from build123d import *

# Parameters (mm, degrees)
F0_R     = 12.5
F2_DEPTH = 236.5
F4_DEPTH = 4


with BuildPart() as f2:
    # F0 (on Right) → F2 (new body, symmetric)
    with BuildSketch(Plane.YZ):
        Circle(F0_R)
    extrude(amount=F2_DEPTH, both=True)

    # F3 (on offset) → F4 (cut)
    with BuildSketch(Plane.XY.offset(12.5)):
        with BuildLine():
            ThreePointArc((-136.5, 4), (-140.5, 0), (-136.5, -4))
            Line((-136.5, -4), (-101.5, -4))
            ThreePointArc((-101.5, -4), (-97.5, 0), (-101.5, 4))
            Line((-101.5, 4), (-136.5, 4))
        make_face()
        with BuildLine():
            ThreePointArc((103.5, 4), (99.5, 0), (103.5, -4))
            Line((103.5, -4), (138.5, -4))
            ThreePointArc((138.5, -4), (142.5, 0), (138.5, 4))
            Line((138.5, 4), (103.5, 4))
        make_face()
    extrude(amount=-F4_DEPTH, mode=Mode.SUBTRACT)


solid = f2.part
Work out the finished part from the listing and answer in its coordinate system (mm). Round coordinates to 2 decimals unless told otherwise and drop trailing zeros. Order: outer loops, then holes, each group sorted by start corner. A loop starts at its lowest first (then second) coordinate and runs counter-clockwise, first axis right, second up. Notation, with made-up numbers: M 4.25,-40 L 39.25,-40 A22 ccw 39.25,-7 Z; hole C 26,59.25 d8. An arc over 180 degrees is marked long. One line per item, written item: value.
Q1. Find section A-A on y = 0. Write down the section's boundary in (x, z), then the cut area to 3 significant figures.
Derived:
outline: M -236.5,-12.5 L 236.5,-12.5 L 236.5,12.5 L 142.5,12.5 L 142.5,8.5 L 99.5,8.5 L 99.5,12.5 L -97.5,12.5 L -97.5,8.5 L -140.5,8.5 L -140.5,12.5 L -236.5,12.5 Z
area: 11,500 mm²
Q2. Determine the mould class of faces 1 (the face through (236.5, 0, 0)), 2 (the face through (3.31, 5.77, -11.09)), 3 (the face through (-119, 0, 8.5)), 4 (the face through (121, 0, 8.5)) for opening direction Y: released by +Y, released by -Y, zero draft, split by the parting line, or undercut.
Derived:
face 1: zero draft
face 2: split by the parting line
face 3: undercut
face 4: undercut
Q3. Find section C-C on z = -7.25. Write down the section's boundary in (x, y), then the cut area to 3 significant figures.
Derived:
outline: M -236.5,-10.18 L 236.5,-10.18 L 236.5,10.18 L -236.5,10.18 Z
area: 9,630 mm²
Q4. Straight lines are drawn through the part: line 1 (Y direction, x = 109.5, z = 10.75); line 2 (Y direction, x = 180.5, z = -1); line 3 (Y direction, x = 212.5, z = 2.5). For each, find the intervals that lie inside material, in ascending order.
Derived:
line 1: -6.38 to -4, 4 to 6.38
line 2: -12.46 to 12.46
line 3: -12.25 to 12.25
Q5. Find section B-B on x = -182. Write down the section's boundary in (y, z), then the cut area to 3 significant figures.
Derived:
outline: C 0,0 d25
area: 491 mm²
Q6. Flat-ended cylindrical pins translate along their axes: pin 1 (9 mm diameter, centred on x = 116, y = -1.5, fed in from +Z); pin 2 (12 mm diameter, centred on x = 169.5, z = -8, fed in from +Y); pin 3 (2 mm diameter, centred on x = -0.5, y = -3, fed in from +Z). Find the tip coordinate at first contact, or state that the pin passes through.
Derived:
pin 1: z = 11.84
pin 2: y = 12.34
pin 3: z = 12.34
